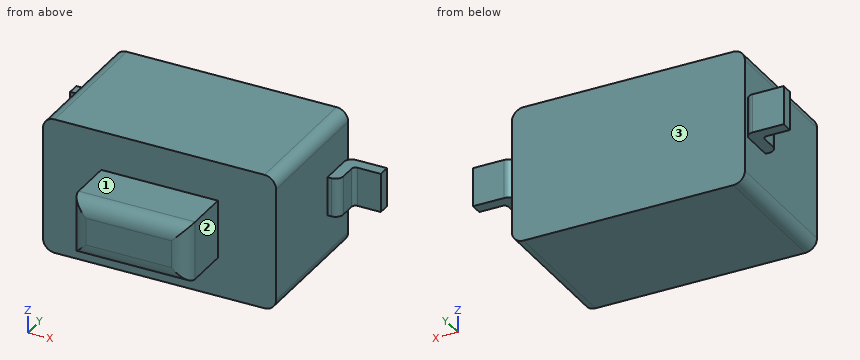
from build123d import *

# Parameters (mm, degrees)
F0_W     = 6
F0_H     = 3.5
F1_DEPTH = 3.5
F2_W     = 3
F2_H     = 1.5
F3_DEPTH = 1.5
F4_R     = 0.3
F5_R     = 0.4
F8_DEPTH = 0.5


# Not quite as in the source:
# - a pattern or mirror of a feature is missing from the dataset's text; its kind, count and spacing are read off the source's solid


with BuildPart() as f1:
    # F0 (on Front) → F1 (new body)
    with BuildSketch(Plane.XZ):
        with Locations((3, 1.75)):
            Rectangle(F0_W, F0_H)
    extrude(amount=F1_DEPTH)

    # F2 (on face) → F3 (join)
    with BuildSketch(Plane.XZ.offset(3.5)):
        with Locations((3, 1.75)):
            Rectangle(F2_W, F2_H)
    extrude(amount=F3_DEPTH)

    # F4
    f4_edges = [f1.edges().sort_by_distance(p)[0] for p in [
        (0, -1.75, 0),
        (0, -1.75, 3.5),
        (6, -1.75, 0),
        (6, -1.75, 3.5),
    ]]
    fillet(f4_edges, radius=F4_R)

    # F5
    f5_edges = [f1.edges().sort_by_distance(p)[0] for p in [
        (1.5, -5, 1.75),
        (3, -5, 2.5),
        (3, -5, 1),
        (4.5, -5, 1.75),
    ]]
    fillet(f5_edges, radius=F5_R)

    # F7 (on mid) → F8 (join, symmetric)
    with BuildSketch(Plane.XY.offset(1.75)):
        with BuildLine():
            Line((-0.1, -1), (0, -1))
            Line((0, -1), (0, -0.2))
            ThreePointArc((0, -0.2), (-0.0585786438, -0.0585786438), (-0.2, 0))
            Line((-0.2, 0), (-1, 0))
            Line((-1, 0), (-1, -0.3))
            Line((-1, -0.3), (-0.4, -0.3))
            ThreePointArc((-0.4, -0.3), (-0.3292893219, -0.3292893219), (-0.3, -0.4))
            Line((-0.3, -0.4), (-0.3, -0.8))
            ThreePointArc((-0.3, -0.8), (-0.2414213562, -0.9414213562), (-0.1, -1))
        make_face()
    f8 = extrude(amount=F8_DEPTH, both=True)

    # F8_copies: F8 across plane
    add(f8.mirror(Plane(origin=(3, 0, 0), x_dir=(0, 0, 1), z_dir=(1, 0, 0))))


solid = f1.part
Can you work these out from the model? Positions are in its coordinate system, mm. Face numbers are marked on the shaded views. A direction names the side the tool comes from. Coordinates: 2 decimals unless noted, no trailing zeros. Write each loop counter-clockwise with the first axis right and the second up, starting at its lowest first coordinate (ties: lowest second). Pieces come first, ordered by that corner, then holes. Notation, with made-up numbers: (50, -22.5) -> (59, -22.5) arc R13 ccw to (59, -16.5) -> close; hole circle Ø10 at (38, -19.75). An arc over 180 degrees is marked (long way). Write item = value, one per line.
(1) Imagine slicing it at D-D (y = -2.9). Please give me the cut outline in (x, z), and give its area (3 significant figures).
Verdict:
outline = (0, 0.3) arc R0.3 ccw to (0.3, 0) -> (5.7, 0) arc R0.3 ccw to (6, 0.3) -> (6, 3.2) arc R0.3 ccw to (5.7, 3.5) -> (0.3, 3.5) arc R0.3 ccw to (0, 3.2) -> close
area = 20.9 mm^2
(2) Imagine slicing it at B-B (z = 1.6). Please give me the cut outline in (x, y), and give its area (3 significant figures).
Verdict:
outline = (-1, -0.3) -> (-0.4, -0.3) arc R0.1 cw to (-0.3, -0.4) -> (-0.3, -0.8) arc R0.2 ccw to (-0.1, -1) -> (0, -1) -> (0, -3.5) -> (1.5, -3.5) -> (1.5, -4.6) arc R0.4 ccw to (1.9, -5) -> (4.1, -5) arc R0.4 ccw to (4.5, -4.6) -> (4.5, -3.5) -> (6, -3.5) -> (6, -1) -> (6.1, -1) arc R0.2 ccw to (6.3, -0.8) -> (6.3, -0.4) arc R0.1 cw to (6.4, -0.3) -> (7, -0.3) -> (7, 0) -> (6.2, 0) arc R0.2 ccw to (6, -0.2) -> (6, 0) -> (0, 0) -> (0, -0.2) arc R0.2 ccw to (-0.2, 0) -> (-1, 0) -> close
area = 26.4 mm^2
(3) If I drill on probe 1 along X at (y, z) = (-1.9, 0.4); probe 2 along Y at (x, z) = (0.5, 2.9); probe 3 along Y at (x, z) = (6.5, 2), over which ranges is the centre line in solid material (lowest first)?
Verdict:
probe_1 = 0 to 6
probe_2 = -3.5 to 0
probe_3 = -0.3 to 0
(4) For pin 1 (0.9 mm diameter, centred on y = -1.5, z = 2, fed in from -X); pin 2 (0.5 mm diameter, centred on x = 6.5, y = -0.5, fed in from -Z); pin 3 (0.8 mm diameter, centred on x = -0.5, y = -0.5, fed in from +Z), each with a flat end and sliding along its axis, tell me the tip position at first contact or that it passes through.
Verdict:
pin_1 = 0
pin_2 = 1.25
pin_3 = 2.25
(5) Imagine slicing it at A-A (y = -0.7). Please give me the cut outline in (x, z), and give its area (3 significant figures).
Verdict:
outline = (-0.3, 1.25) -> (0, 1.25) -> (0, 0.3) arc R0.3 ccw to (0.3, 0) -> (5.7, 0) arc R0.3 ccw to (6, 0.3) -> (6, 1.25) -> (6.3, 1.25) -> (6.3, 2.25) -> (6, 2.25) -> (6, 3.2) arc R0.3 ccw to (5.7, 3.5) -> (0.3, 3.5) arc R0.3 ccw to (0, 3.2) -> (0, 2.25) -> (-0.3, 2.25) -> close
area = 21.5 mm^2
(6) On a 3-axis mill with a long thin cutter (end or side, diameter ignored), from which of +Z, -Z, +X, -X, +Y, -Y can I reach the whole of each face in a straight line? I mean the marked faces 1, 2 and 3. Say none if no direction works.
Verdict:
face_1 = +Z, +X, -X, -Y
face_2 = +Z, -Z, +X, -Y
face_3 = +Z, -Z, +X, -X, +Y
(7) Imagine slicing it at C-C (x = 3.75). Please give me the cut outline in (y, z).
Verdict:
outline = (-5, 1.4) arc R0.4 ccw to (-4.6, 1) -> (-3.5, 1) -> (-3.5, 0) -> (0, 0) -> (0, 3.5) -> (-3.5, 3.5) -> (-3.5, 2.5) -> (-4.6, 2.5) arc R0.4 ccw to (-5, 2.1) -> close
